```python
from build123d import *
from build123d import SkipClean  # not in build123d's __all__

# Parameters (mm, degrees)
F1_DEPTH = 6


# Not quite as in the source:
# - a pattern or mirror of a feature is missing from the dataset's text; its kind, count and spacing are read off the source's solid


with BuildPart() as f1:
    # F0 (on Top) → F1 (new body)
    with BuildSketch(Plane.XY):
        with BuildLine():
            Line((11, 0), (16, 0))
            ThreePointArc((16, 0), (15.1274260959, 5.2116196823), (12.6048775359, 9.854798948))
            ThreePointArc((12.6048775359, 9.854798948), (12.6039156913, 9.856029081), (12.6029537267, 9.8572591203))
            Line((12.6029537267, 9.8572591203), (16.5472631752, 16.6890034859))
            Line((16.5472631752, 16.6890034859), (17.413288579, 16.1890034859))
            add(Edge.make_bspline(
                [(17.413288579, 16.1890034859), (17.5041916061, 16.8045773234), (17.7045445822, 19.4085508868), (15.5298067399, 25.2595570372), (12.9266999082, 31.0960374777), (7.9390301641, 36.5896284217), (5.2735054472, 37.9125925094), (3.8379400503, 38.5036543012)],
                knots=[0, 0, 0, 0, 0.1468390725, 0.3630340887, 0.5865738984, 0.8170443021, 1, 1, 1, 1], degree=3))
            Line((3.8379400503, 38.5036543012), (3.8379400503, 36.3024744126))
            Line((3.8379400503, 36.3024744126), (2.5230119528, 36.3024744126))
            Line((2.5230119528, 36.3024744126), (0, 38.5036543012))
            Line((0, 38.5036543012), (-2.5230119528, 36.3024744126))
            Line((-2.5230119528, 36.3024744126), (-3.8379400503, 36.3024744126))
            Line((-3.8379400503, 36.3024744126), (-3.8379400503, 38.5036543012))
            add(Edge.make_bspline(
                [(-17.413288579, 16.1890034859), (-17.5041916061, 16.8045773234), (-17.7045445822, 19.4085508868), (-15.5298067399, 25.2595570372), (-12.9266999082, 31.0960374777), (-7.9390301641, 36.5896284217), (-5.2735054472, 37.9125925094), (-3.8379400503, 38.5036543012)],
                knots=[0, 0, 0, 0, 0.1468390725, 0.3630340887, 0.5865738984, 0.8170443021, 1, 1, 1, 1], degree=3))
            Line((-17.413288579, 16.1890034859), (-16.5472631752, 16.6890034859))
            Line((-16.5472631752, 16.6890034859), (-12.6029537267, 9.8572591203))
            ThreePointArc((-12.6029537267, 9.8572591203), (-12.6039156913, 9.856029081), (-12.6048775359, 9.854798948))
            ThreePointArc((-12.6048775359, 9.854798948), (-15.1274260959, 5.2116196823), (-16, 0))
            Line((-16, 0), (-11, 0))
            ThreePointArc((-11, 0), (0, 11), (11, 0))
        make_face()
        with BuildLine():
            ThreePointArc((-2.5, 31.9088473916), (0, 34.4088473916), (2.5, 31.9088473916))
            add(Edge.make_bspline(
                [(2.5, 31.9088473916), (2.4331220889, 30.6490394363), (2.4535157828, 30.0127263526), (2.8986373466, 23.7894092903), (6.9226723271, 20.1849518953), (7.2970524444, 20.0978087891), (9.3067939396, 18.8178154736)],
                knots=[0, 0, 0, 0, 0.191959096, 0.4953854958, 0.7661719362, 1, 1, 1, 1], degree=3))
            ThreePointArc((9.3067939396, 18.8178154736), (10.2567995477, 15.4836064725), (6.9615764655, 14.4061255414))
            ThreePointArc((6.9615764655, 14.4061255414), (0, 16), (-6.9615764655, 14.4061255414))
            ThreePointArc((-6.9615764655, 14.4061255414), (-10.2567995477, 15.4836064725), (-9.3067939396, 18.8178154736))
            add(Edge.make_bspline(
                [(-2.5, 31.9088473916), (-2.4331220889, 30.6490394363), (-2.4535157828, 30.0127263526), (-2.8986373466, 23.7894092903), (-6.9226723271, 20.1849518953), (-7.2970524444, 20.0978087891), (-9.3067939396, 18.8178154736)],
                knots=[0, 0, 0, 0, 0.191959096, 0.4953854958, 0.7661719362, 1, 1, 1, 1], degree=3))
        make_face(mode=Mode.SUBTRACT)
    extrude(amount=F1_DEPTH)

    # F1_copies: F1 across plane


with BuildPart() as f1_1:
    add(f1.part, clean=False)
    with SkipClean():  # cleaning this boolean's faces spoils the solid; the shape is the same uncleaned
        add(f1.part.mirror(Plane(origin=(0, 0, 0), x_dir=(0, 0, -1), z_dir=(0, -1, 0))), clean=False)


solid = f1_1.part
```
Input: part model. Units: mm. Frame: model coordinates. A direction names the side the tool comes from. Coordinates: 2 decimals unless noted, no trailing zeros. Order: outer loops, then holes, each group sorted by start corner. A loop starts at its lowest first (then second) coordinate and runs counter-clockwise, first axis right, second up. Notation, with made-up numbers: (2, -17.75) - (6, -17.75) arc R20 ccw to (6, -3.75) - close; hole circle Ø5 at (43, 4.5). An arc over 180 degrees is marked (long way). Put each result on its own line as item: value.
1. Reachability of faces 1 (the face through (-3.838, 37, 3)), 2 (the face through (0, 16, 3)), 3 (the face through (3, -36.302, 3)) from +Z, -Z, +X, -X, +Y, -Y: full face, straight path, thin tool, end or side. Return the list, or none.
Report:
face 1: +Z, -Z, +Y
face 2: +Z, -Z
face 3: +Z, -Z, -Y
2. Contact query for flat-ended pins moving along their axis: pin 1 Ø1.1 at (x, z) = (-3.5, 1.5) entering from +Y; pin 2 Ø2 at (y, z) = (6.5, 1) entering from +X (3 decimals); pin 3 Ø3 at (x, z) = (-4.5, 2.5) entering from -Y; pin 4 Ø1.1 at (y, z) = (-38, 2.5) entering from -X. Output: stop coordinate, or through.
Report:
pin 1: stops at y = 38.5
pin 2: stops at x = 15.025
pin 3: stops at y = -38.5
pin 4: stops at x = -6.05
3. Draft query along X for faces 4 (the face through (3.838, -37, 3)), 5 (the face through (8, -9, 0)). Return one class per face: pulls with the +X half, pulls with the -X half, needs draft (parallel to the pull), parting line crosses it, or undercut.
Report:
face 4: undercut
face 5: needs draft
4. Cut plane A-A on y = 7. Return the cut outline in (x, z), then the cut area to 3 significant figures.
Report:
outline: (-14.39, 0) - (-8.49, 0) - (-8.49, 6) - (-14.39, 6) - close; (8.49, 0) - (14.39, 0) - (14.39, 6) - (8.49, 6) - close
area: 70.8 mm2
5. Line query: line 1 along Y through (x, z) = (0, 5.75); line 2 along X through (y, z) = (0, 3.85); line 3 along Y through (x, z) = (-3.5, 4.25). Output: solid intervals per line, ascending.
Report:
line 1: y = -38.5 to -34.41, -16 to -11, 11 to 16, 34.41 to 38.5
line 2: x = -16 to -11, 11 to 16
line 3: y = -36.3 to -24.39, -15.61 to -10.43, 10.43 to 15.61, 24.39 to 36.3
6. Cut plane B-B on x = 1. Return the cut outline in (y, z), then the cut area to 3 significant figures.
Report:
outline: (-37.63, 0) - (-34.2, 0) - (-34.2, 6) - (-37.63, 6) - close; (-15.97, 0) - (-10.95, 0) - (-10.95, 6) - (-15.97, 6) - close; (10.95, 0) - (15.97, 0) - (15.97, 6) - (10.95, 6) - close; (34.2, 0) - (37.63, 0) - (37.63, 6) - (34.2, 6) - close
area: 101 mm2
7. Cut plane C-C on z = 1.75. State how many separate pieces and enclosed holes the cut face has, then the cut area to 3 significant figures.
Report:
separate pieces: 1
enclosed holes: 3
area: 1,380 mm2
